```python
from build123d import *
from build123d.topology import SkipClean

# Parameters (mm, degrees)
SKETCH1_W               = 170
SKETCH1_H               = 140
BOSS_EXTRUDE1_DEPTH     = 4
BOSS_EXTRUDE2_DEPTH     = 10
CUT_EXTRUDE3_DEPTH      = 221.671701856
CUT_EXTRUDE3_DEPTH_BACK = 221.671701856
CUT_EXTRUDE6_DEPTH      = 10


with BuildPart() as part:
    # Sketch1 → Boss-Extrude1 (new body)
    with BuildSketch(Plane(origin=(0, 0, 0), x_dir=(1, 0, 0), z_dir=(0, 1, 0))):
        with Locations((85, 70)):
            Rectangle(SKETCH1_W, SKETCH1_H)
    extrude(amount=BOSS_EXTRUDE1_DEPTH)

    # Sketch2 → Boss-Extrude2 (add)
    with BuildSketch(Plane(origin=(0, 4, 0), x_dir=(1, 0, 0), z_dir=(0, 1, 0))):
        with BuildLine():
            Line((127.071067812, 127.071067812), (112.928932188, 112.928932188))
            ThreePointArc((112.928932188, 112.928932188), (109.6846987, 110.761204675), (105.857864376, 110))
            Line((105.857864376, 110), (0, 110))
            Line((0, 110), (0, 95))
            Line((0, 95), (94.092172608, 95))
            ThreePointArc((94.092172608, 95), (95.939931673, 93.765366865), (95.50638617, 91.585786438))
            Line((95.50638617, 91.585786438), (86.849531921, 82.928932188))
            ThreePointArc((86.849531921, 82.928932188), (83.605298432, 80.761204675), (79.778464109, 80))
            Line((79.778464109, 80), (30.446951372, 80))
            Line((30.446951372, 80), (0, 80))
            Line((0, 80), (0, 74.5))
            Line((0, 74.5), (80, 74.5))
            ThreePointArc((80, 74.5), (82, 72.5), (80, 70.5))
            Line((80, 70.5), (0, 70.5))
            Line((0, 70.5), (0, 67))
            Line((0, 67), (80, 67))
            ThreePointArc((80, 67), (82, 65), (80, 63))
            Line((80, 63), (0, 63))
            Line((0, 63), (0, 59.5))
            Line((0, 59.5), (80, 59.5))
            ThreePointArc((80, 59.5), (82, 57.5), (80, 55.5))
            Line((80, 55.5), (0, 55.5))
            Line((0, 55.5), (0, 52))
            Line((0, 52), (80, 52))
            ThreePointArc((80, 52), (82, 50), (80, 48))
            Line((80, 48), (0, 48))
            Line((0, 48), (0, 44.5))
            Line((0, 44.5), (80, 44.5))
            ThreePointArc((80, 44.5), (82, 42.5), (80, 40.5))
            Line((80, 40.5), (0, 40.5))
            Line((0, 40.5), (0, 37))
            Line((0, 37), (80, 37))
            ThreePointArc((80, 37), (82, 35), (80, 33))
            Line((80, 33), (0, 33))
            Line((0, 33), (0, 27.5))
            Line((0, 27.5), (88.357864376, 27.5))
            ThreePointArc((88.357864376, 27.5), (92.1846987, 26.738795325), (95.428932188, 24.571067812))
            Line((95.428932188, 24.571067812), (107.071067812, 12.928932188))
            ThreePointArc((107.071067812, 12.928932188), (110.3153013, 10.761204675), (114.142135624, 10))
            Line((114.142135624, 10), (150, 10))
            ThreePointArc((150, 10), (157.071067812, 12.928932188), (160, 20))
            Line((160, 20), (160, 120))
            ThreePointArc((160, 120), (157.071067812, 127.071067812), (150, 130))
            Line((150, 130), (134.142135624, 130))
            ThreePointArc((134.142135624, 130), (130.3153013, 129.238795325), (127.071067812, 127.071067812))
        make_face()
    extrude(amount=BOSS_EXTRUDE2_DEPTH)

    # Sketch4 → Cut-Extrude3 (cut, two sides: drawn at the far end of the back side and taken through both)
    with SkipClean():  # the faces are left unmerged after this step: merging them gives an invalid solid
        with BuildSketch(Plane(origin=(0, 0, 0), x_dir=(1, 0, 0), z_dir=(0, 1, 0)).offset(-CUT_EXTRUDE3_DEPTH_BACK)):
            with BuildLine():
                Line((94.092172608, 95), (0, 95))
                Line((0, 95), (0, 80))
                Line((0, 80), (30.446951372, 80))
                Line((30.446951372, 80), (79.778464109, 80))
                ThreePointArc((79.778464109, 80), (83.605298432, 80.761204675), (86.849531921, 82.928932188))
                Line((86.849531921, 82.928932188), (95.50638617, 91.585786438))
                ThreePointArc((95.50638617, 91.585786438), (95.939931673, 93.765366865), (94.092172608, 95))
            make_face()
        extrude(amount=CUT_EXTRUDE3_DEPTH + CUT_EXTRUDE3_DEPTH_BACK, mode=Mode.SUBTRACT)
    add(part.part.scale(1), mode=Mode.REPLACE)  # the faces are merged on a copy

    # Sketch5 → Cut-Extrude6 (cut)
    with BuildSketch(Plane(origin=(0, 0, 0), x_dir=(1, 0, 0), z_dir=(0, 1, 0))):
        with BuildLine():
            Line((-80, 70.5), (80, 70.5))
            ThreePointArc((80, 70.5), (82, 72.5), (80, 74.5))
            Line((80, 74.5), (-80, 74.5))
            ThreePointArc((-80, 74.5), (-82, 72.5), (-80, 70.5))
        make_face()
        with BuildLine():
            Line((80, 63), (-80, 63))
            ThreePointArc((-80, 63), (-82, 65), (-80, 67))
            Line((-80, 67), (80, 67))
            ThreePointArc((80, 67), (82, 65), (80, 63))
        make_face()
        with BuildLine():
            Line((-80, 55.5), (80, 55.5))
            ThreePointArc((80, 55.5), (82, 57.5), (80, 59.5))
            Line((80, 59.5), (-80, 59.5))
            ThreePointArc((-80, 59.5), (-82, 57.5), (-80, 55.5))
        make_face()
        with BuildLine():
            Line((-80, 48), (80, 48))
            ThreePointArc((80, 48), (82, 50), (80, 52))
            Line((80, 52), (-80, 52))
            ThreePointArc((-80, 52), (-82, 50), (-80, 48))
        make_face()
        with BuildLine():
            Line((-80, 40.5), (80, 40.5))
            ThreePointArc((80, 40.5), (82, 42.5), (80, 44.5))
            Line((80, 44.5), (-80, 44.5))
            ThreePointArc((-80, 44.5), (-82, 42.5), (-80, 40.5))
        make_face()
        with BuildLine():
            Line((-80, 33), (80, 33))
            ThreePointArc((80, 33), (82, 35), (80, 37))
            Line((80, 37), (-80, 37))
            ThreePointArc((-80, 37), (-82, 35), (-80, 33))
        make_face()
    extrude(amount=CUT_EXTRUDE6_DEPTH, mode=Mode.SUBTRACT)


solid = part.part
```
Check sheet for the modelled part. Datum: model origin and axes. Units: mm. A direction names the side the tool comes from. Round coordinates to 2 decimals unless told otherwise and drop trailing zeros. Loops run counter-clockwise (first coordinate to the right, second up) from the corner with the lowest first, then second, coordinate; pieces in that order, holes last. Notation, with made-up numbers: (48, -27) -> (102, -27) arc R10 cw to (102, -10) -> close; hole circle Ø11 at (78, -20.5). An arc over 180 degrees is marked (long way). Answer in a Markdown table with one row per item.
Q1. Sectioned sample at B-B on z = -106. Enter the section's corners in (x, y).
Data:
| item | result |
|---|---|
| outline | (0, 0) -> (170, 0) -> (170, 4) -> (160, 4) -> (160, 14) -> (0, 14) -> close |
Q2. Sectioned sample at D-D on z = -42.5. Enter the section's corners in (x, y), then the cut area to 3 significant figures.
Data:
| item | result |
|---|---|
| outline | (82, 0) -> (170, 0) -> (170, 4) -> (160, 4) -> (160, 14) -> (82, 14) -> close |
| area | 1,130 mm^2 |
Q3. Sectioned sample at A-A on x = 136. Enter the section's corners in (y, z), then the cut area to 3 significant figures.
Data:
| item | result |
|---|---|
| outline | (0, -140) -> (4, -140) -> (4, -130) -> (14, -130) -> (14, -10) -> (4, -10) -> (4, 0) -> (0, 0) -> close |
| area | 1,760 mm^2 |
Q4. Set-up check for faces 1 (the face through (110.265, 8.93, -10.782)), 2 (the face through (114, 14, -71)), 3 (the face through (130.37, 8.93, -129.26)), 4 (the face through (156.99, 8.93, -12.85)), 5 (the face through (41, 7, -52)): record each of +Z, -Z, +X, -X, +Y, -Y from which the full face is reachable in a straight line by a thin tool's end or side.
Data:
| item | result |
|---|---|
| face 1 | +Z, -X, +Y |
| face 2 | +Z, -Z, +X, -X, +Y |
| face 3 | -Z, -X, +Y |
| face 4 | +Z, +X, +Y |
| face 5 | -X, +Y, -Y |
Q5. Thickness scan on L1, parallel to Z at x = 100, y = 7.25; L2, parallel to X at y = 8.25, z = -40; L3, parallel to Z at x = 94, y = 10. Record the ranges inside material, lowest first.
Data:
| item | result |
|---|---|
| L1 | z = -110 to -20 |
| L2 | x = 0 to 160 |
| L3 | z = -110 to -95, -90.08 to -25.76 |
Q6. Sectioned sample at C-C on x = 49.5. Give the number of separate pieces and of enclosed holes in the cut face, then the cut area to 3 significant figures.
Data:
| item | result |
|---|---|
| separate pieces | 8 |
| enclosed holes | 0 |
| area | 839 mm^2 |
Q7. Go/stop test with flat-tipped pins: P1, Ø4, axis at x = 52.5, y = 6.5, coming from the +Z side; P2, Ø1.5, axis at x = 117, y = 12.5, coming from the +Z side; P3, Ø2, axis at y = 11.5, z = -93.5, coming from the +X side. Record where each tip stops, or that it passes through.
Data:
| item | result |
|---|---|
| P1 | stops at z = -27.5 |
| P2 | stops at z = -10 |
| P3 | stops at x = 160 |
